```python
from build123d import *

# Parameters (mm, degrees)
SKETCH1_W           = 48.2
SKETCH1_H           = 26.25
SKETCH1_R           = 1.5
SKETCH1_R_2         = 2
BOSS_EXTRUDE1_DEPTH = 11
BOSS_EXTRUDE2_DEPTH = 2.5
SKETCH3_W           = 8
SKETCH3_H           = 8
CUT_EXTRUDE1_DEPTH  = 30.564769997
FILLET1_R           = 1.5
CUT_EXTRUDE2_DEPTH  = 5
FILLET2_R           = 2


with BuildPart() as part:
    # Sketch1 → Boss-Extrude1 (new body)
    with BuildSketch(Plane(origin=(0, 0, 0), x_dir=(1, 0, 0), z_dir=(0, 1, 0))):
        Rectangle(SKETCH1_W, SKETCH1_H)
        with Locations(Location((-15.1, 8.125, 0), (0, 0, 270))):
            Circle(SKETCH1_R, mode=Mode.SUBTRACT)
        with Locations(Location((15.1, -8.125, 0), (0, 0, 270))):
            Circle(SKETCH1_R, mode=Mode.SUBTRACT)
        with Locations(Location((-15.1, -8.125, 0), (0, 0, 270))):
            Circle(SKETCH1_R_2, mode=Mode.SUBTRACT)
        with Locations(Location((15.1, 8.125, 0), (0, 0, 270))):
            Circle(SKETCH1_R_2, mode=Mode.SUBTRACT)
    extrude(amount=BOSS_EXTRUDE1_DEPTH)

    # Sketch2 → Boss-Extrude2 (add)
    with BuildSketch(Plane(origin=(0, 11, 0), x_dir=(1, 0, 0), z_dir=(0, 1, 0))):
        Polygon((-24.1, -6.125), (-22.1, -6.125), (-22.1, -11.125), (-14.1, -11.125), (-14.1, -13.125), (-24.1, -13.125), align=None)
        Polygon((14.1, 13.125), (14.1, 11.125), (22.1, 11.125), (22.1, 6.125), (24.1, 6.125), (24.1, 13.125), align=None)
    extrude(amount=BOSS_EXTRUDE2_DEPTH)

    # Sketch3 → Cut-Extrude1 (cut, through all)
    with BuildSketch(Plane(origin=(0, 11, 0), x_dir=(1, 0, 0), z_dir=(0, 1, 0))):
        with Locations((-4.63, -9.125)):
            Rectangle(SKETCH3_W, SKETCH3_H)
    extrude(amount=-CUT_EXTRUDE1_DEPTH, mode=Mode.SUBTRACT)

    # Fillet1
    fillet1_edges = [part.edges().sort_by_distance(p)[0] for p in [
        (-8.63, 5.5, 5.125),
        (-0.63, 5.5, 5.125),
    ]]
    fillet(fillet1_edges, radius=FILLET1_R)

    # Sketch5 → Cut-Extrude2 (cut)
    with BuildSketch(Plane.XZ):
        Polygon((-17.85, -9.71271324), (-17.85, -13.125), (-12.35, -13.125), (-12.35, -9.71271324), (-12.35, -6.53728676), (-15.1, -4.949573519), (-17.85, -6.53728676), align=None)
        Polygon((15.1, 4.949573519), (17.85, 6.53728676), (17.85, 9.71271324), (17.85, 13.125), (12.35, 13.125), (12.35, 9.71271324), (12.35, 6.53728676), align=None)
    extrude(amount=-CUT_EXTRUDE2_DEPTH, mode=Mode.SUBTRACT)

    # Fillet2
    fillet2_edges = [part.edges().sort_by_distance(p)[0] for p in [
        (-12.35, 2.5, -13.125),
        (-17.85, 2.5, -13.125),
        (12.35, 2.5, 13.125),
        (17.85, 2.5, 13.125),
    ]]
    fillet(fillet2_edges, radius=FILLET2_R)


solid = part.part
```
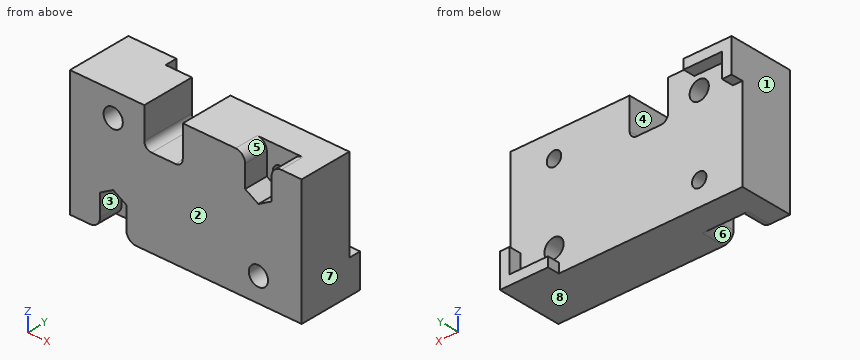
The model under review builds one solid part; all positions refer to its coordinate system, in mm. Face numbers are marked on the shaded views. A direction names the side the tool comes from. Round coordinates to 2 decimals unless told otherwise and drop trailing zeros. Order: outer loops, then holes, each group sorted by start corner. A loop starts at its lowest first (then second) coordinate and runs counter-clockwise, first axis right, second up.
Item 1: Add section A-A, the plane y = 12. State the section outline as (x, z) points (3 decimals).
Working result:
outline: (-24.1, 6.125) - (-22.1, 6.125) - (-22.1, 11.125) - (-14.1, 11.125) - (-14.1, 13.125) - (-24.1, 13.125) - close; (14.1, -13.125) - (24.1, -13.125) - (24.1, -6.125) - (22.1, -6.125) - (22.1, -11.125) - (14.1, -11.125) - close
Item 2: Add section D-D, the plane y = 2.75. State the section outline as (x, z) points (3 decimals).
Working result:
outline: (-24.1, -13.125) - (-19.85, -13.125) arc R2 ccw to (-17.85, -11.125) - (-17.85, -6.537) - (-15.1, -4.95) - (-12.35, -6.537) - (-12.35, -11.125) arc R2 ccw to (-10.35, -13.125) - (24.1, -13.125) - (24.1, 13.125) - (19.85, 13.125) arc R2 ccw to (17.85, 11.125) - (17.85, 6.537) - (15.1, 4.95) - (12.35, 6.537) - (12.35, 11.125) arc R2 ccw to (10.35, 13.125) - (-0.63, 13.125) - (-0.63, 6.625) arc R1.5 cw to (-2.13, 5.125) - (-7.13, 5.125) arc R1.5 cw to (-8.63, 6.625) - (-8.63, 13.125) - (-24.1, 13.125) - close; hole circle Ø4 at (-15.1, 8.125); hole circle Ø4 at (15.1, -8.125)
Item 3: To check wall thickness, follow probe 1 along X at (y, z) = (9, 7); probe 2 along X at (y, z) = (1.75, 9.5); probe 3 along X at (y, z) = (1.75, 5.5). State the ranges of each line that lie inside material, in increasing order.
Working result:
probe 1: x = -24.1 to -16.75, -13.45 to -8.63, -0.63 to 14.11, 16.09 to 24.1
probe 2: x = -24.1 to -16.55, -13.65 to -8.63, -0.63 to 12.35, 17.85 to 24.1
probe 3: x = -24.1 to -8.12, -1.14 to 14.15, 16.05 to 24.1
Item 4: For pin 1 (1 mm diameter, centred on y = 12, z = 12.5, fed in from +X); pin 2 (2.5 mm diameter, centred on x = -15.1, z = -8.125, fed in from -Y); pin 3 (0.6 mm diameter, centred on x = 23, y = 12.5, fed in from +Z) (3 decimals); pin 4 (5.5 mm diameter, centred on x = -5.5, y = 5, fed in from +Z), all flat-tipped, find the tip position at first contact; note any pin that passes through.
Working result:
pin 1: stops at x = -14.1
pin 2: passes through
pin 3: stops at z = -6.125
pin 4: stops at z = 5.63
Item 5: Add section B-B, the plane y = 6.5. State the section outline as (x, z) points (3 decimals), and give its area (3 significant figures).
Working result:
outline: (-24.1, -13.125) - (24.1, -13.125) - (24.1, 13.125) - (-0.63, 13.125) - (-0.63, 6.625) arc R1.5 cw to (-2.13, 5.125) - (-7.13, 5.125) arc R1.5 cw to (-8.63, 6.625) - (-8.63, 13.125) - (-24.1, 13.125) - close; hole circle Ø4 at (-15.1, 8.125); hole circle Ø3 at (-15.1, -8.125); hole circle Ø4 at (15.1, -8.125); hole circle Ø3 at (15.1, 8.125)
area: 1,160 mm2
Item 6: Add section C-C, the plane x = -16. State the section outline as (y, z) points (3 decimals).
Working result:
outline: (0, -5.469) - (5, -5.469) - (5, -6.925) - (11, -6.925) - (11, 6.339) - (0, 6.339) - close; (0, 9.911) - (11, 9.911) - (11, 11.125) - (13.5, 11.125) - (13.5, 13.125) - (0, 13.125) - close; (5, -13.125) - (11, -13.125) - (11, -9.325) - (5, -9.325) - close
Item 7: Machinability: for the marked faces 4, 5, 6, 7 and 8, which of the approach directions +Z, -Z, +X, -X, +Y, -Y give a long, thin tool a straight path to every point of the face, cutting with its end or side? Answer none if there is none.
Working result:
face 4: +Z, +Y, -Y
face 5: +Z, -Y
face 6: -Z, -Y
face 7: +Z, -Z, +X, +Y, -Y
face 8: -Z, +X, -X, +Y, -Y
Item 8: Draft analysis for pull direction X (two halves, no side actions). For the marked faces 1, 2 and 3, state which applies: released by +X, released by -X, zero draft, split by the parting line, or undercut.
Working result:
face 1: released by -X
face 2: zero draft
face 3: undercut
